```python
from build123d import *

# Parameters (mm, degrees)
SKETCH1_R           = 0.8875
BOSS_EXTRUDE1_DEPTH = 2.5


with BuildPart() as part:
    # Sketch1 → Boss-Extrude1 (new body)
    with BuildSketch(Plane.XY):
        with BuildLine():
            Line((0.414365521, 2.024043391), (4.164365521, 2.024043391))
            Line((4.164365521, 2.024043391), (4.164365521, -5.475956609))
            Line((4.164365521, -5.475956609), (0.414365521, -5.475956609))
            ThreePointArc((0.414365521, -5.475956609), (-3.335634479, -1.725956609), (0.414365521, 2.024043391))
        make_face()
        Circle(SKETCH1_R, mode=Mode.SUBTRACT)
        with Locations((0.828731042, -3.451913217)):
            Circle(SKETCH1_R, mode=Mode.SUBTRACT)
    extrude(amount=BOSS_EXTRUDE1_DEPTH)


solid = part.part
```
Part model, mm, in its own coordinate system. Give positions to 0.01 mm unless a question says otherwise; leave off trailing zeros. Write each loop counter-clockwise with the first axis right and the second up, starting at its lowest first coordinate (ties: lowest second). Pieces come first, ordered by that corner, then holes. Notation, with made-up numbers: (16.5, 21) -> (75.5, 21) arc R16 ccw to (75.5, 43) -> close; hole circle Ø8 at (40, 79). An arc over 180 degrees is marked (long way). Put each result on its own line as item: value. Start each with the question number.
Item 1: Wall check: L1, parallel to Y at x = 0.75, z = 2.25; L2, parallel to X at y = -3, z = 1.25; L3, parallel to X at y = -3.5, z = 1.65. Give the ranges that are in metal, low to high. Write a range as [from, to].
Item 2: Cut at A-A (y = 0). List the corners of the cut face in (x, z).
Item 3: Cut at D-D (x = -2). List the corners of the cut face in (y, z), then the cut area to 3 significant figures.
Item 4: Pull direction Y, two halves, no side cores. Call faces 1 (the face through (2, 2.024, 1)), 2 (the face through (2, -5.476, 1)), 3 (the face through (-0.12, 0.88, 1.23)): pulls with the +Y half, pulls with the -Y half, needs draft (parallel to the pull), parting line crosses it, or undercut.
Item 5: Cut at B-B (z = 1.9). State how many separate pieces and enclosed holes the cut face has, then the cut area to 3 significant figures.
Item 6: Pin check, flat tip, straight feed: pin 1 Ø1 at (y, z) = (-1, 1.5) entering from -X. Stop position of the tip, or through.
Item 7: Cut at C-C (y = -3). List the corners of the cut face in (x, z), then the cut area to 3 significant figures.
Answer list:
1. L1: y = [-5.48, -4.34], [-2.57, -0.47], [0.47, 2.02]
1. L2: x = [-3.11, 0.06], [1.59, 4.16]
1. L3: x = [-2.89, -0.06], [1.71, 4.16]
2. outline: (-2.91, 0) -> (-0.89, 0) -> (-0.89, 2.5) -> (-2.91, 2.5) -> close; (0.89, 0) -> (4.16, 0) -> (4.16, 2.5) -> (0.89, 2.5) -> close
3. outline: (-4.6, 0) -> (1.14, 0) -> (1.14, 2.5) -> (-4.6, 2.5) -> close
3. area: 14.3 mm2
4. face 1: pulls with the +Y half
4. face 2: pulls with the -Y half
4. face 3: undercut
5. separate pieces: 1
5. enclosed holes: 2
5. area: 45.3 mm2
6. pin 1: stops at x = -3.33
7. outline: (-3.11, 0) -> (0.06, 0) -> (0.06, 2.5) -> (-3.11, 2.5) -> close; (1.59, 0) -> (4.16, 0) -> (4.16, 2.5) -> (1.59, 2.5) -> close
7. area: 14.4 mm2
